from build123d import *

# Parameters (mm, degrees)
BOSS_EXTRUDE1_DEPTH   = 0.2
BOSS_EXTRUDE1_2_DEPTH = 0.2


with BuildPart() as part:
    # Model → Boss-Extrude1 (new body)
    with BuildSketch(Plane.XY):
        Polygon((-0.719000633, 4.476263641), (-0.709000633, 4.470263641), (4.284999367, 0.831263641), (4.318999367, 0.792263641), (4.379999367, 0.686263641), (4.389999367, 0.663263641), (4.416999367, 0.582263641), (4.422999367, 0.527263641), (4.406999367, 0.404263641), (4.403999367, 0.386263641), (4.265999367, -0.104736359), (4.305999367, -0.454736359), (4.538999367, -0.881736359), (4.549999367, -0.909736359), (4.651999367, -1.300736359), (4.655999367, -1.329736359), (4.665999367, -1.755736359), (4.660999367, -1.792736359), (4.411999367, -2.642736359), (4.392999367, -2.682736359), (3.913999367, -3.323736359), (3.895999367, -3.343736359), (3.418999367, -3.753736359), (3.390999367, -3.771736359), (2.990999367, -3.962736359), (2.937999367, -3.974736359), (2.421999367, -3.974736359), (2.371999367, -3.964736359), (1.865999367, -3.744736359), (1.605999367, -3.664736359), (1.195999367, -3.734736359), (0.876999367, -4.101736359), (0.851999367, -4.123736359), (0.202999367, -4.556736359), (0.143999367, -4.577736359), (-1.991000633, -4.754736359), (-1.997000633, -4.754736359), (-6.627000633, -4.754736359), (-6.660000633, -4.749736359), (-7.143000633, -4.613736359), (-7.197000633, -4.581736359), (-7.814000633, -3.964736359), (-7.999000633, -3.964736359), (-8.005000633, -3.962736359), (-24.783000633, -3.962736359), (-24.850000633, -3.942736359), (-24.896000633, -3.890736359), (-24.907000633, -3.838736359), (-24.907000633, -1.889736359), (-24.888000633, -1.822736359), (-24.835000633, -1.776736359), (-24.783000633, -1.765736359), (-8.005000633, -1.765736359), (-8.004000633, -1.764736359), (-8.004000633, -0.023736359), (-7.984000633, 0.043263641), (-7.970000633, 0.061263641), (-7.541000633, 0.516263641), (-7.480000633, 0.551263641), (-7.450000633, 0.555263641), (-5.694000633, 0.555263641), (-4.897000633, 1.160263641), (-4.832000633, 1.185263641), (-4.822000633, 1.185263641), (-3.674000633, 1.185263641), (-3.284000633, 1.465263641), (-1.099000633, 4.405263641), (-1.063000633, 4.438263641), (-1.011000633, 4.469263641), (-0.952000633, 4.486263641), (-0.787000633, 4.493263641), align=None)
    extrude(amount=BOSS_EXTRUDE1_DEPTH)


with BuildPart() as body_2:
    # Model → Boss-Extrude1 2 (new body)
    with BuildSketch(Plane.XY):
        Polygon((-12.208000633, 15.583263641), (-12.129000633, 15.567263641), (-12.085000633, 15.549263641), (-12.028000633, 15.511263641), (-11.994000633, 15.477263641), (-11.957000633, 15.420263641), (-11.938000633, 15.376263641), (-11.922000633, 15.297263641), (-11.920000633, 15.273263641), (-11.920000633, 14.001263641), (-11.922000633, 13.977263641), (-11.938000633, 13.898263641), (-11.957000633, 13.854263641), (-11.994000633, 13.797263641), (-12.028000633, 13.763263641), (-12.085000633, 13.725263641), (-12.129000633, 13.707263641), (-12.208000633, 13.691263641), (-12.232000633, 13.689263641), (-12.403000633, 13.689263641), (-12.518000633, 13.666263641), (-12.615000633, 13.601263641), (-12.680000633, 13.504263641), (-12.703000633, 13.389263641), (-12.703000633, 10.112263641), (-12.705000633, 10.088263641), (-12.721000633, 10.009263641), (-12.739000633, 9.964263641), (-12.777000633, 9.908263641), (-12.811000633, 9.874263641), (-12.868000633, 9.836263641), (-12.912000633, 9.818263641), (-12.991000633, 9.802263641), (-13.015000633, 9.800263641), (-14.285000633, 9.800263641), (-14.361000633, 9.784263641), (-14.426000633, 9.741263641), (-14.470000633, 9.676263641), (-14.485000633, 9.600263641), (-14.485000633, 9.081263641), (-14.487000633, 9.057263641), (-14.495000633, 9.017263641), (-14.514000633, 8.972263641), (-14.530000633, 8.948263641), (-14.564000633, 8.914263641), (-14.566000633, 8.913263641), (-14.632000633, 8.892263641), (-14.635000633, 8.892263641), (-18.652000633, 8.895263641), (-18.720000633, 8.914263641), (-18.755000633, 8.950263641), (-18.770000633, 8.972263641), (-18.789000633, 9.017263641), (-18.797000633, 9.057263641), (-18.799000633, 9.081263641), (-18.799000633, 9.600263641), (-18.815000633, 9.676263641), (-18.858000633, 9.741263641), (-18.923000633, 9.784263641), (-18.999000633, 9.800263641), (-19.007000633, 9.800263641), (-19.021000633, 9.804263641), (-21.430000633, 9.804263641), (-21.497000633, 9.823263641), (-21.543000633, 9.876263641), (-21.554000633, 9.928263641), (-21.554000633, 9.985263641), (-21.577000633, 10.100263641), (-21.642000633, 10.197263641), (-21.739000633, 10.262263641), (-21.854000633, 10.285263641), (-22.082000633, 10.285263641), (-22.106000633, 10.287263641), (-22.146000633, 10.296263641), (-22.191000633, 10.314263641), (-22.215000633, 10.330263641), (-22.249000633, 10.364263641), (-22.265000633, 10.388263641), (-22.284000633, 10.433263641), (-22.292000633, 10.473263641), (-22.294000633, 10.497263641), (-22.294000633, 12.473263641), (-22.292000633, 12.497263641), (-22.284000633, 12.537263641), (-22.265000633, 12.582263641), (-22.249000633, 12.606263641), (-22.215000633, 12.640263641), (-22.191000633, 12.656263641), (-22.146000633, 12.675263641), (-22.106000633, 12.683263641), (-22.082000633, 12.685263641), (-21.854000633, 12.685263641), (-21.739000633, 12.708263641), (-21.642000633, 12.773263641), (-21.577000633, 12.870263641), (-21.554000633, 12.985263641), (-21.554000633, 15.273263641), (-21.552000633, 15.297263641), (-21.536000633, 15.376263641), (-21.517000633, 15.420263641), (-21.480000633, 15.477263641), (-21.446000633, 15.511263641), (-21.389000633, 15.549263641), (-21.345000633, 15.567263641), (-21.266000633, 15.583263641), (-21.242000633, 15.585263641), (-12.232000633, 15.585263641), align=None)
    extrude(amount=BOSS_EXTRUDE1_2_DEPTH)


solid = part.part
Can you work these out from the model? Positions are in its coordinate system, mm. Give positions to 0.01 mm unless a question says otherwise; leave off trailing zeros. Order: outer loops, then holes, each group sorted by start corner. A loop starts at its lowest first (then second) coordinate and runs counter-clockwise, first axis right, second up. Notation, with made-up numbers: (36.5, -16) - (81.5, -16) arc R25 ccw to (81.5, 23) - close; hole circle Ø3 at (-33.5, -3). An arc over 180 degrees is marked (long way). Write each question's results on one line, items separated by ' | '.
1) Suppose I cut it at A-A, the plane y = 3. Write out the boundary of the cut face in (x, z), then the cut area to 3 significant figures.
Final values:
outline: (-2.14, 0) - (1.31, 0) - (1.31, 0.2) - (-2.14, 0.2) - close | area: 0.690 mm^2
2) Please list where these lines run through material, in increasing order: line 1 along Y through (x, z) = (-4.75, 0.15); line 2 along X through (y, z) = (-1.5, 0.1); line 3 along Y through (x, z) = (-17, 0.1). Write a range as [from, to].
Final values:
line 1: y = [-4.75, 1.19] | line 2: x = [-8, 4.66] | line 3: y = [-3.96, -1.77]
3) Suppose I cut it at B-B, the plane x = -14.25. Write out the boundary of the cut face in (y, z).
Final values:
outline: (-3.96, 0) - (-1.77, 0) - (-1.77, 0.2) - (-3.96, 0.2) - close
